```python
from build123d import *

# Parameters (mm, degrees)
F0_W     = 480
F0_H     = 340
F1_DEPTH = 1970
F2_W     = 380
F2_H     = 50
F3_DEPTH = 350
F2_H_2   = 380
F2_H_3   = 270
F4_DEPTH = 300
F5_W     = 240
F5_H     = 50
F6_DEPTH = 895


with BuildPart() as f1:
    # F0 (on Top) → F1 (new body)
    with BuildSketch(Plane.XY):
        with Locations((-240, 170)):
            Rectangle(F0_W, F0_H)
    extrude(amount=F1_DEPTH)

    # F2 (on face) → F3 (cut)
    with BuildSketch(Plane.XZ):
        with Locations((-240, 25)):
            Rectangle(F2_W, F2_H)
    extrude(amount=-F3_DEPTH, mode=Mode.SUBTRACT)

    # F2 (on face) → F4 (cut)
    with BuildSketch(Plane.XZ):
        with Locations((-240, 290)):
            Rectangle(F2_W, F2_H_2)
        with Locations((-240, 633)):
            Rectangle(F2_W, F2_H_3)
        with Locations((-240, 921)):
            Rectangle(F2_W, F2_H_3)
        with Locations((-240, 1209)):
            Rectangle(F2_W, F2_H_3)
        with Locations((-240, 1497)):
            Rectangle(F2_W, F2_H_3)
        with Locations((-240, 1785)):
            Rectangle(F2_W, F2_H_3)
    extrude(amount=-F4_DEPTH, mode=Mode.SUBTRACT)

    # F5 (on face) → F6 (cut)
    with BuildSketch(Plane(origin=(-480, 0, 0), x_dir=(0, -1, 0), z_dir=(-1, 0, 0))):
        with Locations((-170, 25)):
            Rectangle(F5_W, F5_H)
    extrude(amount=-F6_DEPTH, mode=Mode.SUBTRACT)


solid = f1.part
```
Model file for the job. Use its own axes, mm. A direction names the side the tool comes from. Round coordinates to 2 decimals unless told otherwise and drop trailing zeros. Order: outer loops, then holes, each group sorted by start corner. A loop starts at its lowest first (then second) coordinate and runs counter-clockwise, first axis right, second up. Notation, with made-up numbers: M 52.25,55.25 L 88.25,55.25 A8 ccw 88.25,64.25 Z; hole C 8,33.25 d3. An arc over 180 degrees is marked long. Use CSV: the item, a comma, the result in double quotes.
Item 1: Saw through at B-B (z = 830.5). List the corners of the cut face in (x, y).
Worked answers:
outline,"M -480,0 L -430,0 L -430,300 L -50,300 L -50,0 L 0,0 L 0,340 L -480,340 Z"
Item 2: Pin check, flat tips, straight feed: pin 1 (5 mm diameter, centred on x = -82, y = 304.5, fed in from -Z); pin 2 (5 mm diameter, centred on x = -148, z = 960, fed in from -Y). Stop position of each tip, or through.
Worked answers:
pin 1,"z = 50"
pin 2,"y = 300"
Item 3: Probe probe 1 along X at (y, z) = (95.5, 1583); probe 2 along Y at (x, z) = (-56, 1676); probe 3 along Z at (x, y) = (-243, 315). List the from-to ranges inside material, lowest first.
Worked answers:
probe 1,"-480 to -430, -50 to 0"
probe 2,"300 to 340"
probe 3,"50 to 1970"
Item 4: Saw through at C-C (x = -159). List the corners of the cut face in (y, z).
Worked answers:
outline,"M 0,50 L 340,50 L 340,1970 L 0,1970 L 0,1920 L 300,1920 L 300,1650 L 0,1650 L 0,1632 L 300,1632 L 300,1362 L 0,1362 L 0,1344 L 300,1344 L 300,1074 L 0,1074 L 0,1056 L 300,1056 L 300,786 L 0,786 L 0,768 L 300,768 L 300,498 L 0,498 L 0,480 L 300,480 L 300,100 L 0,100 Z"
Item 5: Saw through at A-A (y = 112). List the corners of the cut face in (x, z).
Worked answers:
outline,"M -480,50 L 0,50 L 0,1970 L -480,1970 Z; hole M -430,100 L -50,100 L -50,480 L -430,480 Z; hole M -430,498 L -50,498 L -50,768 L -430,768 Z; hole M -430,786 L -50,786 L -50,1056 L -430,1056 Z; hole M -430,1074 L -50,1074 L -50,1344 L -430,1344 Z; hole M -430,1362 L -50,1362 L -50,1632 L -430,1632 Z; hole M -430,1650 L -50,1650 L -50,1920 L -430,1920 Z"
Item 6: Pull direction Z, two halves, no side cores. Call faces 3 (the face through (-243, 148, 1344)), 4 (the face through (-430, 315, 25)), 5 (the face through (-243, 148, 1650)), 6 (the face through (-25, 315, 0)): released by +Z, released by -Z, zero draft, split by the parting line, or undercut.
Worked answers:
face 3,"undercut"
face 4,"zero draft"
face 5,"undercut"
face 6,"released by -Z"
Item 7: Which spindle directions (+Z, -Z, +X, -X, +Y, -Y) get a long thin tool onto all of the face, cutting with end or side? Do faces 1 (the face through (-455, 290, 25)), 2 (the face through (-50, 148, 1783)). Say none if no direction does.
Worked answers:
face 1,"-Z, +X, -X"
face 2,"-Y"
